Part model, mm, in its own coordinate system. Face numbers are marked on the shaded views. A direction names the side the tool comes from. Round coordinates to 2 decimals unless told otherwise and drop trailing zeros. Write each loop counter-clockwise with the first axis right and the second up, starting at its lowest first coordinate (ties: lowest second). Pieces come first, ordered by that corner, then holes. Notation, with made-up numbers: (-13.5, 28.5) -> (-1.5, 28.5) arc R14 cw to (-1.5, 53.5) -> close; hole circle Ø11 at (-27, 3.5). An arc over 180 degrees is marked (long way). Return JSON: item names as keys, results as strings. Group by question number.
(1) Drop flat-ended pins along their axis: pin 1 Ø1 at (y, z) = (-2, 54) entering from -X; pin 2 Ø3.5 at (x, z) = (-6, 60) entering from +Y (3 decimals); pin 3 Ø10 at (x, z) = (-58, 8) entering from +Y (3 decimals); pin 4 Ø18 at (x, z) = (-37, 41) entering from -Y (3 decimals). Give the stop position or say it passes through.
(2) Drill centre lines: L1, parallel to Y at x = -37.5, z = 66; L2, parallel to X at y = -2, z = 14.5; L3, parallel to X at y = 9.5, z = 64. Where is each one in solid material? Low to high. Write a range as from..to.
(3) Mould opens along Y. For the marked faces 4, 5, 6 and 7 say: +Y half, -Y half, draft (parallel to the pull), parting line (faces both ways), or undercut.
(4) Tool access for the marked faces 1, 2 and 3: list every direction of +Z, -Z, +X, -X, +Y, -Y with a clear straight run to the whole face (end or side of a thin tool).
(5) Saw through at A-A (z = 33.5). List the corners of the cut face in (x, y).
(6) Saw through at B-B (x = -60.5). List the corners of the cut face in (y, z).
(7) Saw through at C-C (y = -28). List the corners of the cut face in (x, z), plus the area to 3 significant figures.
from build123d import *

# Parameters (mm, degrees)
ESQUISSE1_W             = 110
ESQUISSE1_H             = 90
ESQUISSE1_W_2           = 100
ESQUISSE1_H_2           = 80
BOSS_EXTRU_1_DEPTH      = 5
ESQUISSE1_32_W          = 100
ESQUISSE1_32_H          = 80
ESQUISSE1_32_W_2        = 90
ESQUISSE1_32_H_2        = 70
BOSS_EXTRU_2_DEPTH      = 70
ESQUISSE1_33_W          = 90
ESQUISSE1_33_H          = 70
BOSS_EXTRU_3_DEPTH      = 10
ENL_V_MAT_EXTRU_3_DEPTH = 10
ENL_V_MAT_EXTRU_4_DEPTH = 10
CONG_1_R                = 1
CONG_2_R                = 1


with BuildPart() as part:
    # Esquisse1 → Boss.-Extru.1 (new body)
    with BuildSketch(Plane.XY):
        with Locations((-53.377032771, -27.155018472)):
            Rectangle(ESQUISSE1_W, ESQUISSE1_H)
        with Locations((-53.377032771, -27.155018472)):
            Rectangle(ESQUISSE1_W_2, ESQUISSE1_H_2, mode=Mode.SUBTRACT)
    extrude(amount=BOSS_EXTRU_1_DEPTH)

    # Esquisse1<32> → Boss.-Extru.2 (add)
    with BuildSketch(Plane.XY):
        with Locations((-53.377032771, -27.155018472)):
            Rectangle(ESQUISSE1_32_W, ESQUISSE1_32_H)
        with Locations((-53.377032771, -27.155018472)):
            Rectangle(ESQUISSE1_32_W_2, ESQUISSE1_32_H_2, mode=Mode.SUBTRACT)
    extrude(amount=BOSS_EXTRU_2_DEPTH)

    # Esquisse1<33> → Boss.-Extru.3 (add)
    with BuildSketch(Plane.XY):
        with Locations((-53.377032771, -27.155018472)):
            Rectangle(ESQUISSE1_33_W, ESQUISSE1_33_H)
    extrude(amount=BOSS_EXTRU_3_DEPTH)

    # Esquisse11 → Enlèv. mat.-Extru.3 (cut)
    with BuildSketch(Plane(origin=(-3.377032771, 0, 0), x_dir=(0, 0, -1), z_dir=(1, 0, 0))):
        Polygon((-56.824573519, -7.155018472), (-58.41228676, -4.405018472), (-61.58771324, -4.405018472), (-63.175426481, -7.155018472), (-61.58771324, -9.905018472), (-58.41228676, -9.905018472), align=None)
    extrude(amount=-ENL_V_MAT_EXTRU_3_DEPTH, mode=Mode.SUBTRACT)

    # Esquisse13 → Enlèv. mat.-Extru.4 (cut)
    with BuildSketch(Plane.ZY.offset(103.377032771)):
        Polygon((63.175426481, -47.155018472), (61.58771324, -44.405018472), (58.41228676, -44.405018472), (56.824573519, -47.155018472), (58.41228676, -49.905018472), (61.58771324, -49.905018472), align=None)
    extrude(amount=-ENL_V_MAT_EXTRU_4_DEPTH, mode=Mode.SUBTRACT)

    # Congé1
    cong_1_edges = [part.edges().sort_by_distance(p)[0] for p in [
        (-53.377032771, 12.844981528, 70),
        (-103.377032771, -27.155018472, 70),
        (-53.377032771, -67.155018472, 70),
        (-3.377032771, -27.155018472, 70),
    ]]
    fillet(cong_1_edges, radius=CONG_1_R)

    # Congé2
    cong_2_edges = [part.edges().sort_by_distance(p)[0] for p in [
        (-53.377032771, -72.155018472, 5),
        (1.622967229, -27.155018472, 5),
        (-53.377032771, 17.844981528, 5),
        (-108.377032771, -27.155018472, 5),
    ]]
    fillet(cong_2_edges, radius=CONG_2_R)


solid = part.part
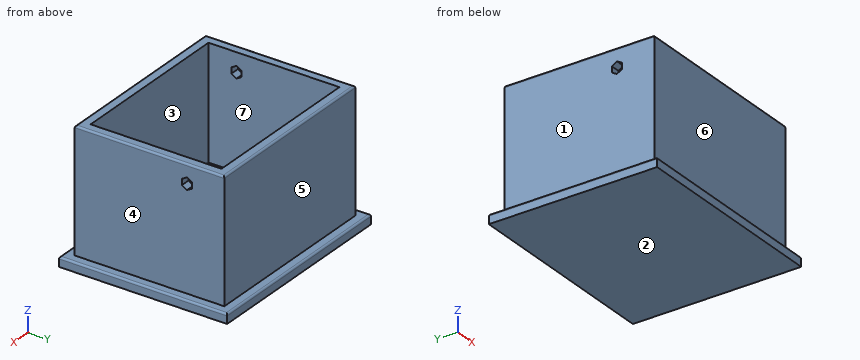
Computed values:
{
 "1": {"pin 1": "x = -103.38", "pin 2": "y = 12.845", "pin 3": "y = 17.845", "pin 4": "y = -67.155"},
 "2": {"L1": "-67.16..-62.16, 7.84..12.84", "L2": "-103.38..-98.38, -8.38..-3.38", "L3": "-103.38..-3.38"},
 "3": {"face 4": "draft", "face 5": "+Y half", "face 6": "-Y half", "face 7": "undercut"},
 "4": {"face 1": "+Z, -X, +Y, -Y", "face 2": "-Z, +X, -X, +Y, -Y", "face 3": "+Z"},
 "5": {"outline": "(-103.38, -67.16) -> (-3.38, -67.16) -> (-3.38, 12.84) -> (-103.38, 12.84) -> close; hole (-98.38, -62.16) -> (-8.38, -62.16) -> (-8.38, 7.84) -> (-98.38, 7.84) -> close"},
 "6": {"outline": "(-72.16, 0) -> (17.84, 0) -> (17.84, 4) arc R1 ccw to (16.84, 5) -> (12.84, 5) -> (12.84, 69) arc R1 ccw to (11.84, 70) -> (7.84, 70) -> (7.84, 10) -> (-62.16, 10) -> (-62.16, 70) -> (-66.16, 70) arc R1 ccw to (-67.16, 69) -> (-67.16, 5) -> (-71.16, 5) arc R1 ccw to (-72.16, 4) -> close"},
 "7": {"outline": "(-108.38, 0) -> (1.62, 0) -> (1.62, 4) arc R1 ccw to (0.62, 5) -> (-3.38, 5) -> (-3.38, 69) arc R1 ccw to (-4.38, 70) -> (-8.38, 70) -> (-8.38, 10) -> (-98.38, 10) -> (-98.38, 70) -> (-102.38, 70) arc R1 ccw to (-103.38, 69) -> (-103.38, 5) -> (-107.38, 5) arc R1 ccw to (-108.38, 4) -> close", "area": "1,650 mm2"}
}
